```python
from build123d import *

# Parameters (mm, degrees)
SKETCH1_R           = 2.5
SKETCH1_W           = 5
SKETCH1_H           = 3.175
BOSS_EXTRUDE1_DEPTH = 3.175


with BuildPart() as part:
    # Sketch1 → Boss-Extrude1 (new body)
    with BuildSketch(Plane.XY):
        Polygon((-147.32, 0), (-106.16, 0), (-106.16, 3.175), (-124.46, 3.175), (-124.46, 13.175), (-22.86, 13.175), (-22.86, 3.175), (-41.16, 3.175), (-41.16, 0), (0, 0), (0, -5), (3.175, -5), (3.175, -10), (0, -10), (0, -15), (3.175, -15), (3.175, -20), (0, -20), (0, -25), (3.175, -25), (3.175, -30), (0, -30), (0, -49.53), (-147.32, -49.53), (-147.32, -30), (-150.495, -30), (-150.495, -25), (-147.32, -25), (-147.32, -20), (-150.495, -20), (-150.495, -15), (-147.32, -15), (-147.32, -10), (-150.495, -10), (-150.495, -5), (-147.32, -5), align=None)
        with Locations((-110.49, -36.83)):
            Circle(SKETCH1_R, mode=Mode.SUBTRACT)
        with Locations((-36.83, -36.83)):
            Circle(SKETCH1_R, mode=Mode.SUBTRACT)
        with Locations((-98.66, 1.5875)):
            Rectangle(SKETCH1_W, SKETCH1_H, mode=Mode.SUBTRACT)
        with Locations((-48.66, 1.5875)):
            Rectangle(SKETCH1_W, SKETCH1_H, mode=Mode.SUBTRACT)
        with Locations((-88.66, 1.5875)):
            Rectangle(SKETCH1_W, SKETCH1_H, mode=Mode.SUBTRACT)
        with Locations((-78.66, 1.5875)):
            Rectangle(SKETCH1_W, SKETCH1_H, mode=Mode.SUBTRACT)
        with Locations((-68.66, 1.5875)):
            Rectangle(SKETCH1_W, SKETCH1_H, mode=Mode.SUBTRACT)
        with Locations((-58.66, 1.5875)):
            Rectangle(SKETCH1_W, SKETCH1_H, mode=Mode.SUBTRACT)
    extrude(amount=BOSS_EXTRUDE1_DEPTH)


solid = part.part
```
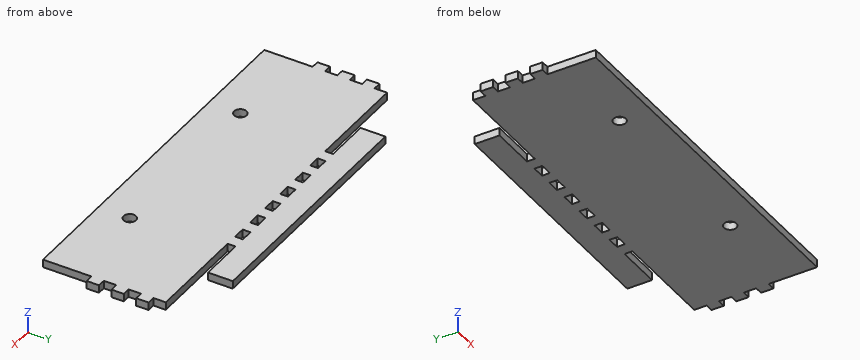
CAD build for the part. Positions are in the model's coordinates, mm. Give positions to 0.01 mm unless a question says otherwise; leave off trailing zeros. Order: outer loops, then holes, each group sorted by start corner. A loop starts at its lowest first (then second) coordinate and runs counter-clockwise, first axis right, second up. Notation, with made-up numbers: M -13,60.25 L 12,60.25 A16 ccw 12,82.25 Z; hole C 83.5,25.25 d8. An arc over 180 degrees is marked long. Put each result on its own line as item: value. Start each with the question number.
(1) Saw through at A-A, the plane y = -36.83. Write the cut outline in (x, z) (3 decimals), then the cut area to 3 significant figures.
(2) Saw through at D-D, the plane y = -13. Write the cut outline in (x, z) (3 decimals).
(3) Saw through at B-B, the plane x = -36.83. Write the cut outline in (y, z) (3 decimals).
(4) Drill centre lines: line 1 along Y through (x, z) = (-36.83, 2.1) (3 decimals); line 2 along Y through (x, z) = (-90.5, 2.15) (3 decimals); line 3 along Y through (x, z) = (-112, 1.2) (3 decimals). Where is each one in solid material? Low to high.
(5) Saw through at C-C, the plane z = 0.85. Give the number of separate pieces and of enclosed holes in the cut face, then the cut area to 3 significant figures.
(6) Flat gauge pins, fed straight in: pin 1 Ø1.6 at (y, z) = (2, 2) entering from -X; pin 2 Ø1.6 at (x, z) = (1, 2) entering from +Y; pin 3 Ø1.6 at (y, z) = (-40.5, 1.5) entering from -X. Where does each tip first touch, or does it go through?
Check result:
1. outline: M -147.32,0 L -112.99,0 L -112.99,3.175 L -147.32,3.175 Z; M -107.99,0 L -39.33,0 L -39.33,3.175 L -107.99,3.175 Z; M -34.33,0 L 0,0 L 0,3.175 L -34.33,3.175 Z
1. area: 436 mm2
2. outline: M -147.32,0 L 0,0 L 0,3.175 L -147.32,3.175 Z
3. outline: M -49.53,0 L -39.33,0 L -39.33,3.175 L -49.53,3.175 Z; M -34.33,0 L 0,0 L 0,3.175 L -34.33,3.175 Z; M 3.175,0 L 13.175,0 L 13.175,3.175 L 3.175,3.175 Z
4. line 1: y = -49.53 to -39.33, -34.33 to 0, 3.175 to 13.175
4. line 2: y = -49.53 to 0, 3.175 to 13.175
4. line 3: y = -49.53 to -38.822, -34.838 to 0, 3.175 to 13.175
5. separate pieces: 1
5. enclosed holes: 8
5. area: 8,480 mm2
6. pin 1: stops at x = -106.16
6. pin 2: stops at y = -5
6. pin 3: stops at x = -147.32
